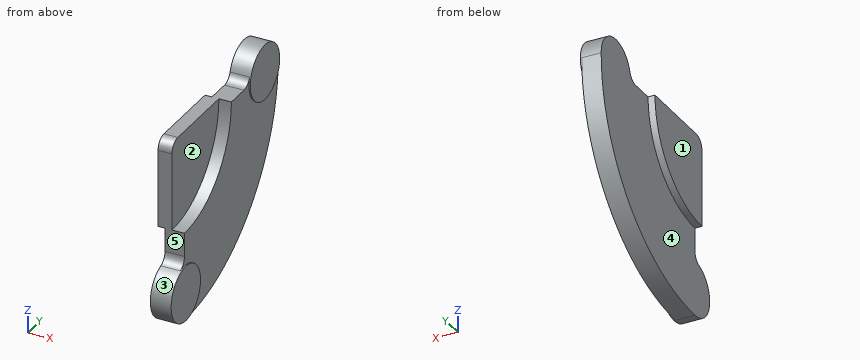
```python
from build123d import *

# Parameters (mm, degrees)
SALIENTE_EXTRUIR1_DEPTH = 2.5
SALIENTE_EXTRUIR2_START = 7
SALIENTE_EXTRUIR2_DEPTH = 7
SALIENTE_EXTRUIR3_START = 7.5
CROQUIS2_4_R            = 10
SALIENTE_EXTRUIR3_DEPTH = 7.5
REDONDEO1_R             = 4
REDONDEO2_R             = 4


with BuildPart() as part:
    # Croquis2 → Saliente-Extruir1 (new, symmetric)
    with BuildSketch(Plane(origin=(0, 0, 0), x_dir=(0, 0, -1), z_dir=(1, 0, 0))):
        with BuildLine():
            ThreePointArc((31.95, 0), (22.592061659, 22.592061659), (0, 31.95))
            Line((0, 31.95), (0, 0))
            Line((0, 0), (31.95, 0))
        make_face()
    extrude(amount=SALIENTE_EXTRUIR1_DEPTH, both=True)

    # Croquis2_3 → Saliente-Extruir2 (add)
    with BuildSketch(Plane(origin=(0, 0, 0), x_dir=(0, 0, -1), z_dir=(1, 0, 0)).offset(SALIENTE_EXTRUIR2_START)):
        with BuildLine():
            ThreePointArc((10, 53.9), (7.071067812, 46.828932188), (0, 43.9))
            Line((0, 43.9), (0, 31.95))
            ThreePointArc((0, 31.95), (22.592061659, 22.592061659), (31.95, 0))
            Line((31.95, 0), (43.9, 0))
            ThreePointArc((43.9, 0), (53.9, 10), (63.9, 0))
            ThreePointArc((63.9, 0), (45.184123318, 45.184123318), (0, 63.9))
            ThreePointArc((0, 63.9), (7.071067812, 60.971067812), (10, 53.9))
        make_face()
    extrude(amount=-SALIENTE_EXTRUIR2_DEPTH)

    # Croquis2_4 → Saliente-Extruir3 (add)
    with BuildSketch(Plane(origin=(0, 0, 0), x_dir=(0, 0, -1), z_dir=(1, 0, 0)).offset(SALIENTE_EXTRUIR3_START)):
        with Locations(Location((0, 53.9, 0), (0, 0, 270))):
            Circle(CROQUIS2_4_R)
        with Locations((53.9, 0)):
            Circle(CROQUIS2_4_R)
    extrude(amount=-SALIENTE_EXTRUIR3_DEPTH)

    # Redondeo1
    redondeo1_edges = [part.edges().sort_by_distance(p)[0] for p in [
        (0, 0, 0),
    ]]
    fillet(redondeo1_edges, radius=REDONDEO1_R)

    # Redondeo2
    # the kernel refuses this fillet: 4 mm, written as the material it adds along each edge
    with BuildSketch(Plane(origin=(7, 0, -43.9), x_dir=(0, 0, 1), z_dir=(-1, 0, 0))) as redondeo2_piece_1:
        with BuildLine():
            CenterArc((3.416407865, -4), REDONDEO2_R, 90, 73.398450401)
            ThreePointArc((-0.416851525, -2.857142857), (-0.104761631, -1.443695821), (0, 0))
            Line((0, 0), (3.416407865, 0))
        make_face()
    extrude(amount=7)
    with BuildSketch(Plane(origin=(7, 43.9, 0), x_dir=(0, -1, 0), z_dir=(-1, 0, 0))) as redondeo2_piece_2:
        with BuildLine():
            CenterArc((3.416407865, 4), REDONDEO2_R, 196.601549599, 73.398450401)
            ThreePointArc((-0.416851525, 2.857142857), (-0.104761631, 1.443695821), (0, 0))
            Line((0, 0), (3.416407865, 0))
        make_face()
    extrude(amount=7)


solid = part.part
```
Work out the finished part from the listing and answer in its coordinate system (mm). Face numbers are marked on the shaded views. A direction names the side the tool comes from. Give positions to 0.01 mm unless a question says otherwise; leave off trailing zeros. Order: outer loops, then holes, each group sorted by start corner. A loop starts at its lowest first (then second) coordinate and runs counter-clockwise, first axis right, second up. Notation, with made-up numbers: (40.5, 33.5) - (89.5, 33.5) arc R18 cw to (89.5, 50.5) - close; hole circle Ø3 at (68, -29). An arc over 180 degrees is marked (long way). One line per item, written item: value. Start each with the question number.
1. Each of these flat-tipped pins is pushed along its axis until it touches: pin 1 Ø4 at (x, y) = (0, 47) entering from +Z; pin 2 Ø1 at (x, y) = (2.5, 21) entering from +Z; pin 3 Ø3 at (x, y) = (6, -2) entering from -Z; pin 4 Ø1.5 at (x, z) = (-1, -39.5) entering from +Y. Where does it stop, or does it pass through?
2. Section A-A, the plane x = 5.5 is taken. Write down the section's boundary in (y, z).
3. Section B-B, the plane z = -30 is taken. Write down the section's boundary in (x, y).
4. Consider line 1 (X direction, y = 40, z = -38.5); line 2 (Z direction, x = 6, y = 55); line 3 (X direction, y = 48.5, z = 5.5). Determine where each line is inside the solid, lowest interval first.
5. Which of the six approach directions +Z, -Z, +X, -X, +Y, -Y give full straight-line access (tool end or side, diameter ignored) to the marked faces 1, 2, 3, 4 and 5?
6. Section D-D, the plane z = -8.5 is taken. Write down the section's boundary in (x, y), then the cut area to 3 significant figures.
7. Section C-C, the plane y = 53.9 is taken. Write down the section's boundary in (x, z).
Filled sheet:
1. pin 1: z = 8.72
1. pin 2: z = 0
1. pin 3: z = -63.89
1. pin 4: through
2. outline: (-2.86, -44.32) arc R10 ccw to (0, -63.9) arc R63.9 ccw to (63.9, 0) arc R10 ccw to (44.32, 2.86) arc R4 cw to (40.48, 0) - (31.95, 0) arc R31.95 cw to (0, -31.95) - (0, -40.48) arc R4 cw to start
3. outline: (-2.5, 0) - (2.5, 0) - (2.5, 10.99) - (7, 10.99) - (7, 56.42) - (0, 56.42) - (0, 10.99) - (-2.5, 10.99) - close
4. line 1: 0 to 7
4. line 2: -32.53 to 9.94
4. line 3: 0 to 7.5
5. face 1: +Z, -Z, -X, +Y, -Y
5. face 2: +Z, +X, -Y
5. face 3: +X
5. face 4: -Z, -X, +Y
5. face 5: +Z, +X, -X, -Y
6. outline: (-2.5, 0) - (2.5, 0) - (2.5, 30.8) - (7, 30.8) - (7, 48.63) - (7.5, 48.63) - (7.5, 59.17) - (7, 59.17) - (7, 63.33) - (0, 63.33) - (0, 30.8) - (-2.5, 30.8) - close
6. area: 387 mm²
7. outline: (0, -34.32) - (7, -34.32) - (7, -10) - (7.5, -10) - (7.5, 10) - (0, 10) - close
